Design review of the part built by this model. Coordinates are the model's own, in mm. A direction names the side the tool comes from. Coordinates: 2 decimals unless noted, no trailing zeros. Loops run counter-clockwise (first coordinate to the right, second up) from the corner with the lowest first, then second, coordinate; pieces in that order, holes last. Notation, with made-up numbers: (11, 54.25) -> (39, 54.25) arc R28 cw to (39, 72.25) -> close; hole circle Ø8 at (-39, 53). An arc over 180 degrees is marked (long way). Answer in a Markdown table with one row per item.
```python
from build123d import *

# Parameters (mm, degrees)
F0_W     = 25
F0_H     = 50
F1_DEPTH = 2
F2_R     = 2.8
F3_R     = 0.4


with BuildPart() as f1:
    # F0 (on Top) → F1 (new body)
    with BuildSketch(Plane.XY):
        Rectangle(F0_W, F0_H)
        Polygon((-10.1, 17.6), (-10.1, 22.6), (-5.1, 22.6), (10.1, 22.6), (10.1, -22.6), (-10.1, -22.6), align=None, mode=Mode.SUBTRACT)
        Polygon((-5.1, 22.6), (-10.1, 22.6), (-10.1, 17.6), align=None)
    extrude(amount=F1_DEPTH)

    # F2
    f2_edges = [f1.edges().sort_by_distance(p)[0] for p in [
        (-12.5, 25, 1),
        (-12.5, -25, 1),
        (12.5, -25, 1),
        (12.5, 25, 1),
    ]]
    fillet(f2_edges, radius=F2_R)

    # F3
    f3_edges = [f1.edges().sort_by_distance(p)[0] for p in [
        (10.1, 22.6, 1),
        (-5.1, 22.6, 1),
        (-10.1, 17.6, 1),
        (-10.1, -22.6, 1),
        (10.1, -22.6, 1),
    ]]
    fillet(f3_edges, radius=F3_R)


solid = f1.part
```
(1) Take a section at C-C on z = 1. Give the boundary of the cut face in (x, y).
Evaluation:
| item | result |
|---|---|
| outline | (-12.5, -22.2) arc R2.8 ccw to (-9.7, -25) -> (9.7, -25) arc R2.8 ccw to (12.5, -22.2) -> (12.5, 22.2) arc R2.8 ccw to (9.7, 25) -> (-9.7, 25) arc R2.8 ccw to (-12.5, 22.2) -> close; hole (-10.1, -22.2) arc R0.4 ccw to (-9.7, -22.6) -> (9.7, -22.6) arc R0.4 ccw to (10.1, -22.2) -> (10.1, 22.2) arc R0.4 ccw to (9.7, 22.6) -> (-4.93, 22.6) arc R0.4 ccw to (-5.22, 22.48) -> (-9.98, 17.72) arc R0.4 ccw to (-10.1, 17.43) -> close |
(2) To check wall thickness, follow probe 1 along X at (y, z) = (2, 1.1); probe 2 along Y at (x, z) = (1.5, 1.85); probe 3 along X at (y, z) = (19, 0.25). State the ranges of each line that lie inside material, in increasing order.
Evaluation:
| item | result |
|---|---|
| probe 1 | x = -12.5 to -10.1, 10.1 to 12.5 |
| probe 2 | y = -25 to -22.6, 22.6 to 25 |
| probe 3 | x = -12.5 to -8.7, 10.1 to 12.5 |
(3) Take a section at B-B on y = -5.5. Give the boundary of the cut face in (x, z).
Evaluation:
| item | result |
|---|---|
| outline | (-12.5, 0) -> (-10.1, 0) -> (-10.1, 2) -> (-12.5, 2) -> close; (10.1, 0) -> (12.5, 0) -> (12.5, 2) -> (10.1, 2) -> close |
(4) Draft analysis for pull direction Y (two halves, no side actions). For faces 1 (the cylindrical face through (-11.7, -24.16, 1.01)), 2 (the flat face through (0, -22.6, 1)), 3 (the flat face through (-11, -2, 2)), 4 (the flat face through (0, 25, 1)), state which applies: pulls with the +Y half, pulls with the -Y half, needs draft (parallel to the pull), parting line crosses it, or undercut.
Evaluation:
| item | result |
|---|---|
| face 1 | pulls with the -Y half |
| face 2 | undercut |
| face 3 | needs draft |
| face 4 | pulls with the +Y half |
(5) Tool access review of faces 5 (the flat face through (2, 22.6, 1)), 6 (the cylindrical face through (11.7, 24.16, 1.01)): name each direction out of +Z, -Z, +X, -X, +Y, -Y from which nothing blocks a thin tool from reaching the whole face with its end or side.
Evaluation:
| item | result |
|---|---|
| face 5 | +Z, -Z |
| face 6 | +Z, -Z, +X, +Y |
(6) Take a section at A-A on x = -7. Give the boundary of the cut face in (y, z), and give its area (3 significant figures).
Evaluation:
| item | result |
|---|---|
| outline | (-25, 0) -> (-22.6, 0) -> (-22.6, 2) -> (-25, 2) -> close; (20.7, 0) -> (25, 0) -> (25, 2) -> (20.7, 2) -> close |
| area | 13.4 mm² |
